```python
from build123d import *

# Parameters (mm, degrees)
SKETCH1_R           = 7.5
BOSS_EXTRUDE1_DEPTH = 6
CHAMFER1_SIZE       = 0.5


with BuildPart() as part:
    # Sketch1 → Boss-Extrude1 (new body)
    with BuildSketch(Plane.XY):
        with BuildLine():
            Line((9.643002644, -1.05), (13.943002644, -1.05))
            Line((13.943002644, -1.05), (13.943002644, 1.05))
            Line((13.943002644, 1.05), (9.643002644, 1.05))
            ThreePointArc((9.643002644, 1.05), (0, 9.7), (-9.643002644, 1.05))
            Line((-9.643002644, 1.05), (-13.943002644, 1.05))
            Line((-13.943002644, 1.05), (-13.943002644, -1.05))
            Line((-13.943002644, -1.05), (-9.643002644, -1.05))
            ThreePointArc((-9.643002644, -1.05), (0, -9.7), (9.643002644, -1.05))
        make_face()
        Circle(SKETCH1_R, mode=Mode.SUBTRACT)
    extrude(amount=BOSS_EXTRUDE1_DEPTH)

    # Chamfer1
    chamfer1_edges = [part.edges().sort_by_distance(p)[0] for p in [
        (0, -9.7, 0),
        (-11.793002644, -1.05, 0),
        (-13.943002644, 0, 0),
        (-11.793002644, 1.05, 0),
        (-11.793002644, -1.05, 6),
        (0, -9.7, 6),
        (11.793002644, -1.05, 6),
        (-7.5, 0, 0),
        (-7.5, 0, 6),
        (13.943002644, 0, 6),
        (11.793002644, 1.05, 6),
        (0, 9.7, 6),
        (-11.793002644, 1.05, 6),
        (0, 9.7, 0),
        (-13.943002644, 0, 6),
        (11.793002644, 1.05, 0),
        (13.943002644, 0, 0),
        (11.793002644, -1.05, 0),
    ]]
    chamfer(chamfer1_edges, length=CHAMFER1_SIZE)


solid = part.part
```
Geometry: final body of the model. Coordinates: model frame, mm. A direction names the side the tool comes from. Coordinates: 2 decimals unless noted, no trailing zeros. Order: outer loops, then holes, each group sorted by start corner. A loop starts at its lowest first (then second) coordinate and runs counter-clockwise, first axis right, second up. Notation, with made-up numbers: M 2,16 L 33,16 A17 ccw 33,39 Z; hole C -17,-33 d7. An arc over 180 degrees is marked long. Answer in a Markdown table with one row per item. Add a question column.
Q1. Contact query for flat-ended pins moving along their axis: P1, Ø10, axis at x = -4.5, y = -2.5, coming from the +Z side; P2, Ø1.3, axis at x = -11.5, z = 2.5, coming from the -Y side; P3, Ø3.5, axis at x = 13, z = 2.5, coming from the +Y side; P4, Ø1, axis at x = 8.5, y = 5.5, coming from the +Z side. Output: stop coordinate, or through.
Q2. Section query A-A on y = 0. Return the cut outline in (x, z), and give its area (3 significant figures).
Q3. Line query: L1, parallel to Y at x = 0.25, z = 3.5; L2, parallel to Y at x = -1.5, z = 2; L3, parallel to X at y = 2.75, z = 3.25. Output: solid intervals per line, ascending.
Q4. Section query B-B on x = 0. Return the cut outline in (y, z), and give its area (3 significant figures).
Q5. Section query C-C on z = 4.75. Return the cut outline in (x, y).
Q6. Reachability of faces 5 (the flat face through (-12, -1.05, 3)), 6 (the flat face through (12, -1.05, 3)), 7 (the flat face through (12, 1.05, 3)), 8 (the cylindrical face through (-0.199, -9.698, 2.965)) from +Z, -Z, +X, -X, +Y, -Y: full face, straight path, thin tool, end or side. Return the list, or none.
Q7. Mould query, pull axis X, two halves, no side actions, for faces 1 (the conical face through (0.197, 9.333, 5.865)), 2 (the flat face through (-12, 1.05, 3)), 3 (the cylindrical face through (-7.493, 0.33, 2.965)), 4 (the flat face through (13.943, 0, 3)). Classes: released by +X, released by -X, zero draft, split by the parting line, or undercut.
Completed:
| question | item | result |
|---|---|---|
| 1 | P1 | stops at z = 6 |
| 1 | P2 | stops at y = -1.05 |
| 1 | P3 | stops at y = 1.05 |
| 1 | P4 | stops at z = 5.58 |
| 2 | outline | M -13.94,0.5 L -13.44,0 L -8,0 L -7.5,0.5 L -7.5,5.5 L -8,6 L -13.44,6 L -13.94,5.5 Z; M 7.5,0.5 L 8,0 L 13.44,0 L 13.94,0.5 L 13.94,5.5 L 13.44,6 L 8,6 L 7.5,5.5 Z |
| 2 | area | 76.3 mm2 |
| 3 | L1 | y = -9.7 to -7.5, 7.5 to 9.7 |
| 3 | L2 | y = -9.58 to -7.35, 7.35 to 9.58 |
| 3 | L3 | x = -9.3 to -6.98, 6.98 to 9.3 |
| 4 | outline | M -9.7,0.5 L -9.2,0 L -8,0 L -7.5,0.5 L -7.5,5.5 L -8,6 L -9.2,6 L -9.7,5.5 Z; M 7.5,0.5 L 8,0 L 9.2,0 L 9.7,0.5 L 9.7,5.5 L 9.2,6 L 8,6 L 7.5,5.5 Z |
| 4 | area | 25.4 mm2 |
| 5 | outline | M -13.94,-1.05 L -9.64,-1.05 A9.7 ccw 9.64,-1.05 L 13.94,-1.05 L 13.94,1.05 L 9.64,1.05 A9.7 ccw -9.64,1.05 L -13.94,1.05 Z; hole C 0,0 d15 |
| 6 | face 5 | +Z, -Z, -X, -Y |
| 6 | face 6 | +Z, -Z, +X, -Y |
| 6 | face 7 | +Z, -Z, +X, +Y |
| 6 | face 8 | +Z, -Z, -Y |
| 7 | face 1 | split by the parting line |
| 7 | face 2 | zero draft |
| 7 | face 3 | undercut |
| 7 | face 4 | released by +X |
